Read the model definition and answer for the solid it produces. Units are mm, in the model's axes. A direction names the side the tool comes from. Give positions to 0.01 mm unless a question says otherwise; leave off trailing zeros. Order: outer loops, then holes, each group sorted by start corner. A loop starts at its lowest first (then second) coordinate and runs counter-clockwise, first axis right, second up. Notation, with made-up numbers: (-21, 83.25) - (24, 83.25) arc R14 ccw to (24, 90.25) - close; hole circle Ø11 at (57, 67). An arc over 180 degrees is marked (long way). Return JSON: item names as keys, results as strings.
```python
from build123d import *

# Parameters (mm, degrees)
EXTRUDE_1_DEPTH     = 10
SKETCH_2_W          = 36.5
SKETCH_2_H          = 10
EXTRUDE_2_DEPTH     = 10
CHAMFER_1_SIZE      = 10
SKETCH_3_R          = 1.6
CUT_EXTRUDE_1_DEPTH = 89.5
SKETCH_4_R          = 1.6
CUT_EXTRUDE_2_DEPTH = 89.5
SKETCH_5_R          = 3
CUT_EXTRUDE_3_DEPTH = 32
SKETCH_6_R          = 3
CUT_EXTRUDE_4_DEPTH = 67


with BuildPart() as part:
    # ｽｹｯﾁ1 → ﾎﾞｽ - 押し出し1 (new body)
    with BuildSketch(Plane.XY):
        Polygon((0, 0), (0, 80), (5, 80), (36.5, 10), (36.5, 0), align=None)
    extrude(amount=EXTRUDE_1_DEPTH)

    # ｽｹｯﾁ2 → ﾎﾞｽ - 押し出し2 (add)
    with BuildSketch(Plane(origin=(0, 0, 0), x_dir=(-1, 0, 0), z_dir=(0, 0, -1))):
        with Locations((-18.25, 5)):
            Rectangle(SKETCH_2_W, SKETCH_2_H)
    extrude(amount=EXTRUDE_2_DEPTH)

    # 面取り1
    chamfer_1_edges = [part.edges().sort_by_distance(p)[0] for p in [
        (18.25, 10, 0),
    ]]
    chamfer(chamfer_1_edges, length=CHAMFER_1_SIZE - 0.0001)  # a hair under: the kernel refuses the full size

    # ｽｹｯﾁ3 → ｶｯﾄ - 押し出し1 (cut, through all)
    with BuildSketch(Plane(origin=(36.5, 0, 0), x_dir=(0, 0, -1), z_dir=(1, 0, 0))):
        with Locations((-5, 5)):
            Circle(SKETCH_3_R)
        with Locations((-5, 75)):
            Circle(SKETCH_3_R)
    extrude(amount=-CUT_EXTRUDE_1_DEPTH, mode=Mode.SUBTRACT)

    # ｽｹｯﾁ4 → ｶｯﾄ - 押し出し2 (cut, through all)
    with BuildSketch(Plane(origin=(0, 0, 0), x_dir=(-1, 0, 0), z_dir=(0, -1, 0))):
        with Locations(Location((-28.9, 5, 0), (0, 0, 180))):
            Circle(SKETCH_4_R)
    extrude(amount=-CUT_EXTRUDE_2_DEPTH, mode=Mode.SUBTRACT)

    # ｽｹｯﾁ5 → ｶｯﾄ - 押し出し3 (cut)
    with BuildSketch(Plane(origin=(36.5, 0, 0), x_dir=(0, 0, -1), z_dir=(1, 0, 0))):
        with Locations((-5, 75)):
            Circle(SKETCH_5_R)
    extrude(amount=-CUT_EXTRUDE_3_DEPTH, mode=Mode.SUBTRACT)

    # ｽｹｯﾁ6 → ｶｯﾄ - 押し出し4 (cut)
    with BuildSketch(Plane(origin=(0, 80, 0), x_dir=(1, 0, 0), z_dir=(0, 1, 0))):
        with Locations((28.9, 5)):
            Circle(SKETCH_6_R)
    extrude(amount=-CUT_EXTRUDE_4_DEPTH, mode=Mode.SUBTRACT)


solid = part.part
```
Q1. A cutting plane is placed at B-B (z = 5). Write down the section's boundary in (x, y).
Values:
{"outline": "(0, 0) - (36.5, 0) - (36.5, 3.4) - (0, 3.4) - close; (0, 6.6) - (36.5, 6.6) - (36.5, 10) - (8.6, 72) - (4.5, 72) - (4.5, 73.4) - (0, 73.4) - close; (0, 76.6) - (4.5, 76.6) - (4.5, 78) - (5.9, 78) - (5, 80) - (0, 80) - close"}
Q2. For faces 1 (the flat face through (19, 5, -10)), 2 (the flat face through (4.5, 73.7, 3.7)), 3 (the flat face through (9, 44, 0)), 4 (the cylindrical face through (29, 15, -2)), determine the directions among +Z, -Z, +X, -X, +Y, -Y from which every point of the face is accessible in a straight line to the end or side of a thin tool.
Values:
{"face 1": "-Z, +X, -X, +Y, -Y", "face 2": "+X", "face 3": "-Z, +X, -X, +Y", "face 4": "+Y"}
Q3. Consider L1, parallel to Z at x = 2.2, y = 75; L2, parallel to Z at x = 7.5, y = 23; L3, parallel to X at y = 14.6, z = -5. Determine where each line is inside the solid, lowest interval first.
Values:
{"L1": "z = 0 to 3.4, 6.6 to 10", "L2": "z = 0 to 10", "L3": "x = 0 to 25.9, 31.9 to 34.43"}
Q4. A cutting plane is placed at A-A (y = 5). Write down the section's boundary in (x, z).
Values:
{"outline": "(0, -10) - (36.5, -10) - (36.5, 3.4) - (0, 3.4) - close; (0, 6.6) - (36.5, 6.6) - (36.5, 10) - (0, 10) - close; hole circle Ø3.2 at (28.9, -5)"}
Q5. Given pin 1 (5.5 mm diameter, centred on x = 30.5, z = -4.5, fed in from +Y); pin 2 (5 mm diameter, centred on x = 9, y = 42, fed in from -Z); pin 3 (1 mm diameter, centred on y = 33.5, z = 5.5, fed in from +X), each flat-ended and moving along its own axis, determine where each tip first touches the part or whether it passes through.
Values:
{"pin 1": "stops at y = 18.25", "pin 2": "stops at z = 0", "pin 3": "stops at x = 26.15"}
Q6. Determine the mould class of faces 5 (the flat face through (36.5, 5, 0)), 6 (the flat face through (14, 32, 10)), 7 (the cylindrical face through (18.51, 4.03, 6.27)) for opening direction Z: released by +Z, released by -Z, zero draft, split by the parting line, or undercut.
Values:
{"face 5": "zero draft", "face 6": "released by +Z", "face 7": "undercut"}
Q7. A cutting plane is placed at D-D (y = 75). Write down the section's boundary in (x, z).
Values:
{"outline": "(0, 0) - (7.25, 0) - (7.25, 2) - (4.5, 2) - (4.5, 3.4) - (0, 3.4) - close; (0, 6.6) - (4.5, 6.6) - (4.5, 8) - (7.25, 8) - (7.25, 10) - (0, 10) - close"}
